from build123d import *

# Parameters (mm, degrees)
SKETCH1_W            = 23.5
SKETCH1_H            = 3.2
BOSS_EXTRUDE1_DEPTH  = 15.8
SKETCH2_R            = 2.4
BOSS_EXTRUDE2_DEPTH  = 1.6
LPATTERN1_COUNT      = 2
LPATTERN1_PITCH      = 8
LPATTERN1_COUNT_DIR2 = 4
LPATTERN1_PITCH_DIR2 = 8
SHELL1_T             = -1.2
SKETCH4_R            = 3.25
SKETCH4_R_2          = 2.4
BOSS_EXTRUDE3_DEPTH  = 1.8
LPATTERN2_COUNT      = 2
LPATTERN2_PITCH      = 8


with BuildPart() as part:
    # Sketch1 → Boss-Extrude1 (new body)
    with BuildSketch(Plane.XY):
        with Locations((11.75, 1.6)):
            Rectangle(SKETCH1_W, SKETCH1_H)
    extrude(amount=-BOSS_EXTRUDE1_DEPTH)

    # Sketch2 → Boss-Extrude2 (add)
    with BuildSketch(Plane(origin=(0, 3.2, 0), x_dir=(1, 0, 0), z_dir=(0, 1, 0))):
        with Locations(Location((3.9, 3.9, 0), (0, 0, 270))):
            Circle(SKETCH2_R)
    boss_extrude2 = extrude(amount=BOSS_EXTRUDE2_DEPTH)

    # LPattern1: Boss-Extrude2 2 × 4, 2 skipped
    with Locations(*[(j * LPATTERN1_PITCH_DIR2, 0, -i * LPATTERN1_PITCH) for i in range(LPATTERN1_COUNT) for j in range(LPATTERN1_COUNT_DIR2) if (i, j) not in ((0, 0), (0, 3), (1, 3))]):
        add(boss_extrude2)

    # Shell1
    shell1_openings = [part.faces().sort_by_distance(p)[0] for p in [
        (11.75, 0, -7.9),
    ]]
    offset(amount=SHELL1_T, openings=shell1_openings, kind=Kind.INTERSECTION)

    # Sketch4 → Boss-Extrude3 (add)
    with BuildSketch(Plane.XZ.offset(-2)):
        with Locations(Location((7.9, -7.9, 0), (0, 0, 90))):
            Circle(SKETCH4_R)
        with Locations(Location((7.9, -7.9, 0), (0, 0, 270))):
            Circle(SKETCH4_R_2, mode=Mode.SUBTRACT)
    boss_extrude3 = extrude(amount=BOSS_EXTRUDE3_DEPTH)

    # LPattern2: Boss-Extrude3 ×2
    with Locations(*[(i * LPATTERN2_PITCH, 0, 0) for i in range(1, LPATTERN2_COUNT)]):
        add(boss_extrude3)


solid = part.part
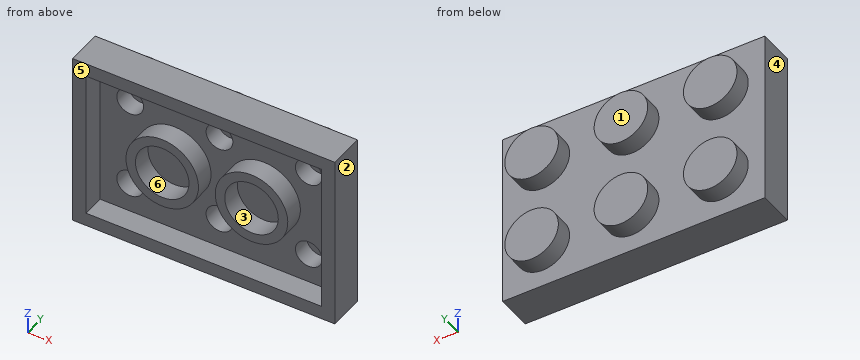
For this review, take the finished solid that the model builds, in its own axes (mm). Face numbers are marked on the shaded views. A direction names the side the tool comes from. Give positions to 0.01 mm unless a question says otherwise; leave off trailing zeros. Order: outer loops, then holes, each group sorted by start corner. A loop starts at its lowest first (then second) coordinate and runs counter-clockwise, first axis right, second up. Notation, with made-up numbers: (-28, -6) - (21, -6) arc R14 cw to (21, 10) - close; hole circle Ø2 at (-22, 39.25). An arc over 180 degrees is marked (long way). Answer as a JSON object with one key per item and string values. Group by question number.
Item 1: Machinability: for the marked faces 5 and 6, which of the approach directions +Z, -Z, +X, -X, +Y, -Y give a long, thin tool a straight path to every point of the face, cutting with its end or side? Answer none if there is none.
Item 2: Wall thickness on line 1 along X through (y, z) = (3, -11.9); line 2 along Z through (x, y) = (11.9, 2.5); line 3 along X through (y, z) = (0.8, -7.9): over which ranges is each line inside the solid? List them lowest first.
Item 3: Take a section at A-A on y = 1.6. Give the boundary of the cut face in (x, z).
Item 4: Draft analysis for pull direction X (two halves, no side actions). For the marked faces 1, 2, 3 and 4, state which applies: pulls with the +X half, pulls with the -X half, needs draft (parallel to the pull), parting line crosses it, or undercut.
Item 5: Take a section at B-B on y = 2.7. Give the boundary of the cut face in (x, z).
Item 6: Take a section at C-C on x = 7.9. Give the boundary of the cut face in (y, z), and give its area (3 significant figures).
Item 7: Clearance check with flat-ended pins moving along their axes: pin 1 Ø3 at (x, z) = (15.5, -8) entering from -Y; pin 2 Ø2.5 at (x, z) = (6.5, -8) entering from -Y; pin 3 Ø6 at (x, z) = (15.9, -7.9) entering from +Y. State where each tip first meets the part, or that it passes through.
Reported:
{
 "1": {"face 5": "+Z, -Z, +X, -X, -Y", "face 6": "-Y"},
 "2": {"line 1": "0 to 2.7, 5.1 to 10.7, 13.1 to 18.7, 21.1 to 23.5", "line 2": "-15.8 to -13.1, -10.7 to -5.1, -2.7 to 0", "line 3": "0 to 1.2, 4.65 to 5.5, 10.3 to 11.15, 12.65 to 13.5, 18.3 to 19.15, 22.3 to 23.5"},
 "3": {"outline": "(0, -15.8) - (23.5, -15.8) - (23.5, 0) - (0, 0) - close; circle Ø6.5 at (7.9, -7.9); circle Ø6.5 at (15.9, -7.9); hole (1.2, -14.6) - (22.3, -14.6) - (22.3, -1.2) - (1.2, -1.2) - close; hole circle Ø4.8 at (7.9, -7.9); hole circle Ø4.8 at (15.9, -7.9)"},
 "4": {"face 1": "needs draft", "face 2": "pulls with the +X half", "face 3": "undercut", "face 4": "pulls with the -X half"},
 "5": {"outline": "(0, -15.8) - (23.5, -15.8) - (23.5, 0) - (0, 0) - close; hole circle Ø2.4 at (3.9, -11.9); hole circle Ø2.4 at (3.9, -3.9); hole circle Ø2.4 at (11.9, -11.9); hole circle Ø2.4 at (11.9, -3.9); hole circle Ø2.4 at (19.9, -11.9); hole circle Ø2.4 at (19.9, -3.9)"},
 "6": {"outline": "(0, -15.8) - (3.2, -15.8) - (3.2, 0) - (0, 0) - (0, -1.2) - (2, -1.2) - (2, -4.65) - (0.2, -4.65) - (0.2, -5.5) - (2, -5.5) - (2, -10.3) - (0.2, -10.3) - (0.2, -11.15) - (2, -11.15) - (2, -14.6) - (0, -14.6) - close", "area": "26.8 mm^2"},
 "7": {"pin 1": "y = 2", "pin 2": "y = 0.2", "pin 3": "y = 3.2"}
}
